Verification items for the finished model (mm, model axes). A direction names the side the tool comes from. Round coordinates to 2 decimals unless told otherwise and drop trailing zeros. Order: outer loops, then holes, each group sorted by start corner. A loop starts at its lowest first (then second) coordinate and runs counter-clockwise, first axis right, second up. Notation, with made-up numbers: M 46.25,26 L 50.25,26 A14 cw 50.25,32 Z; hole C 21,2.25 d8. An arc over 180 degrees is marked long. Use one line per item in the form item = value. Start each with the question number.
Item 1: Cross-section at A-A on x = 22.5. Enter the section's corners in (y, z).
Item 2: Tool access check on faces 1 (the cylindrical face through (-21.06, 3.83, 3.13)), 2 (the cylindrical face through (9.736, 39.768, 7.133)). Record the directions out of +Z, -Z, +X, -X, +Y, -Y that give a thin tool (end or side, any length) a straight path to the whole face; none if there is none.
Item 3: Cross-section at D-D on x = -16. Enter the section's corners in (y, z).
Item 4: Cross-section at C-C on z = 2.75. Count the separate pieces of the cut face and the enclosed holes in it, then the cut area to 3 significant figures.
Item 5: Release check for a two-part mould opening along X. For faces 3 (the flat face through (24.932, 44.733, 3.131)), 4 (the flat face through (0, 0, 3)), 5 (the cylindrical face through (-26.185, 15.859, 3.131)) record: +X half, -X half, draft (parallel to the pull), parting line (faces both ways), or undercut.
Item 6: Thickness scan on probe 1 along Y at (x, z) = (27, 4); probe 2 along Y at (x, z) = (28, 3.25); probe 3 along Z at (x, y) = (23, 11.5). Record the ranges inside material, lowest first. Write a range as [from, to].
Item 7: Cross-section at B-B on y = 43. Enter the section's corners in (x, z).
Item 8: Go/stop test with flat-tipped pins: pin 1 Ø10.5 at (x, y) = (-11.11, 45.97) entering from +Z; pin 2 Ø2 at (y, z) = (41, 1) entering from -X; pin 3 Ø6 at (x, y) = (-13, 23.5) entering from +Z; pin 4 Ø2 at (x, z) = (-14.5, 1) entering from +Y. Record where each tip stops, or that it passes through.
from build123d import *

# Parameters (mm, degrees)
SKETCH1_R           = 3.96875
BOSS_EXTRUDE1_DEPTH = 6.35
SKETCH2_R           = 1.190625
CUT_EXTRUDE1_DEPTH  = 6.35
SKETCH3_R           = 6.35
SKETCH3_R_2         = 3.96875
BOSS_EXTRUDE2_DEPTH = 1.5875


with BuildPart() as part:
    # Sketch1 → Boss-Extrude1 (new body)
    with BuildSketch(Plane.XY):
        Polygon((-25.4, 0), (25.4, 0), (39.320442167, 32.659792071), (10.134148885, 57.15), (-10.134148885, 57.15), (-39.320442167, 32.659792071), align=None)
        with Locations((11.1125, 45.967395581)):
            Circle(SKETCH1_R, mode=Mode.SUBTRACT)
        with Locations((-11.1125, 45.967395581)):
            Circle(SKETCH1_R, mode=Mode.SUBTRACT)
        with Locations((30.570028855, 29.640590295)):
            Circle(SKETCH1_R, mode=Mode.SUBTRACT)
        with Locations((-30.570028855, 29.640590295)):
            Circle(SKETCH1_R, mode=Mode.SUBTRACT)
    extrude(amount=BOSS_EXTRUDE1_DEPTH)

    # Sketch2 → Cut-Extrude1 (cut)
    with BuildSketch(Plane(origin=(0, 0, 0), x_dir=(-1, 0, 0), z_dir=(0, 0, -1))):
        with Locations((-27.374737278, 15.806737027)):
            Circle(SKETCH2_R)
        with Locations((-22.248493734, 3.779673069)):
            Circle(SKETCH2_R)
        with Locations((22.248493734, 3.779673069)):
            Circle(SKETCH2_R)
        with Locations((27.374737278, 15.806737027)):
            Circle(SKETCH2_R)
    extrude(amount=-CUT_EXTRUDE1_DEPTH, mode=Mode.SUBTRACT)

    # Sketch3 → Boss-Extrude2 (add)
    with BuildSketch(Plane.XY.offset(6.35)):
        with Locations((-11.1125, 45.967395581)):
            Circle(SKETCH3_R)
        with Locations((-11.1125, 45.967395581)):
            Circle(SKETCH3_R_2, mode=Mode.SUBTRACT)
        with Locations((11.1125, 45.967395581)):
            Circle(SKETCH3_R)
        with Locations((11.1125, 45.967395581)):
            Circle(SKETCH3_R_2, mode=Mode.SUBTRACT)
        with Locations((-30.570028855, 29.640590295)):
            Circle(SKETCH3_R)
        with Locations((-30.570028855, 29.640590295)):
            Circle(SKETCH3_R_2, mode=Mode.SUBTRACT)
        with Locations((30.570028855, 29.640590295)):
            Circle(SKETCH3_R)
        with Locations((30.570028855, 29.640590295)):
            Circle(SKETCH3_R_2, mode=Mode.SUBTRACT)
    extrude(amount=BOSS_EXTRUDE2_DEPTH)


solid = part.part
Output values:
q1.outline = M 0,0 L 2.62,0 L 2.62,6.35 L 0,6.35 Z; M 4.94,0 L 46.77,0 L 46.77,6.35 L 4.94,6.35 Z
q2.face_1 = +Z, -Z
q2.face_2 = +Z
q3.outline = M 0,0 L 52.23,0 L 52.23,6.35 L 50.02,6.35 L 50.02,7.94 L 41.91,7.94 L 41.91,6.35 L 0,6.35 Z
q4.separate_pieces = 1
q4.enclosed_holes = 8
q4.area = 3,110 mm2
q5.face_3 = +X half
q5.face_4 = draft
q5.face_5 = undercut
q6.probe_1 = [3.75, 14.68], [16.94, 27.91], [31.37, 43]
q6.probe_2 = [6.1, 14.79], [16.82, 26.62], [32.66, 42.16]
q6.probe_3 = [0, 6.35]
q7.outline = M -27,0 L -13.75,0 L -13.75,7.94 L -16.73,7.94 L -16.73,6.35 L -27,6.35 Z; M -8.48,0 L 8.48,0 L 8.48,7.94 L 5.5,7.94 L 5.5,6.35 L -5.5,6.35 L -5.5,7.94 L -8.48,7.94 Z; M 13.75,0 L 27,0 L 27,6.35 L 16.73,6.35 L 16.73,7.94 L 13.75,7.94 Z
q8.pin_1 = 7.94
q8.pin_2 = -30.57
q8.pin_3 = 6.35
q8.pin_4 = 54.33
